from build123d import *

# Parameters (mm, degrees)
SKETCH2_R           = 6.281650674
SKETCH3_R           = 13.256970647
BOSS_EXTRUDE2_DEPTH = 93.98
FILLET1_R           = 5.08


with BuildPart() as part:
    # Sweep1: sweep along a curve in space
    with BuildLine() as sweep1_path:
        Line((-101.863707381, 710.985218526, -786.864459981), (-101.863707381, 710.985218526, -861.202210018))
        ThreePointArc((-101.863707381, 710.985218526, -861.202210018), (-107.071348812, 710.985218526, -873.774568588), (-119.643707381, 710.985218526, -878.982210018))
        Line((-119.643707381, 710.985218526, -878.982210018), (-194.958974291, 710.985218526, -878.982210018))
        ThreePointArc((-194.958974291, 710.985218526, -878.982210018), (-207.531332861, 710.985218526, -884.189851449), (-212.738974291, 710.985218526, -896.762210018))
        Line((-212.738974291, 710.985218526, -896.762210018), (-212.738974291, 710.985218526, -997.376214376))
    # Sketch2 → Sweep1 (sweep)
    with BuildSketch(Plane(origin=(-212.738974291, 710.985218526, -997.376214376), x_dir=(-1, 0, 0), z_dir=(0, 0, -1))):
        Circle(SKETCH2_R)
    sweep(path=sweep1_path.line)

    # Sketch3 → Boss-Extrude2 (add)
    with BuildSketch(Plane(origin=(0, 0, -997.376214376), x_dir=(-1, 0, 0), z_dir=(0, 0, -1))):
        with Locations((212.738974291, 710.985218526)):
            Circle(SKETCH3_R)
    extrude(amount=-BOSS_EXTRUDE2_DEPTH)

    # Fillet1
    fillet1_edges = [part.edges().sort_by_distance(p)[0] for p in [
        (-199.482003644, 710.985218526, -903.396214376),
        (-199.482003644, 710.985218526, -997.376214376),
    ]]
    fillet(fillet1_edges, radius=FILLET1_R)


solid = part.part
Check sheet for the modelled part. Datum: model origin and axes. Units: mm. A direction names the side the tool comes from. Give positions to 0.01 mm unless a question says otherwise; leave off trailing zeros. Order: outer loops, then holes, each group sorted by start corner. A loop starts at its lowest first (then second) coordinate and runs counter-clockwise, first axis right, second up. Notation, with made-up numbers: (64.25, 30.5) - (85.25, 30.5) arc R17 ccw to (85.25, 61.5) - close; hole circle Ø8 at (-11, 14.5). An arc over 180 degrees is marked (long way). Answer as CSV lines item,"result".
1. Scan lines: probe 1 along X at (y, z) = (710.5, -819); probe 2 along Z at (x, y) = (-205, 707.5); probe 3 along X at (y, z) = (714.5, -957). Record each from-to range of solid material in increasing order. Write a range as from..to.
Result sheet:
probe 1,"-108.13..-95.6"
probe 2,"-997.37..-903.41, -889.23..-876.06"
probe 3,"-225.52..-199.96"
2. Go/stop test with flat-tipped pins: P1, Ø8, axis at x = -120, y = 719, coming from the -Z side; P2, Ø6, axis at y = 708.5, z = -972.5, coming from the +X side; P3, Ø1.5, axis at y = 715.5, z = -839, coming from the -X side. Record where each tip stops, or that it passes through.
Result sheet:
P1,"z = -883.81"
P2,"x = -199.48"
P3,"x = -106.89"
3. Section check A-A (z = -972). Record the boundary of the cut face in (x, y).
Result sheet:
outline,"circle Ø26.51 at (-212.74, 710.99)"
4. Tool access check on faces 1 (the face through (-157.83, 708.58, -873.18)), 2 (the face through (-102, 711, -786.864)), 3 (the face through (-107.666, 708.579, -824.554)). Record the directions out of +Z, -Z, +X, -X, +Y, -Y that give a thin tool (end or side, any length) a straight path to the whole face; none if there is none.
Result sheet:
face 1,"none"
face 2,"+Z, +X, -X, +Y, -Y"
face 3,"+Z"
5. Mould release check, pull along Z, two halves, no side actions. Record for faces 4 (the face through (-213, 711, -997.376)), 5 (the face through (-209.865, 698.043, -950.973)), 6 (the face through (-206.463, 711.261, -900.126)): released by +Z, released by -Z, zero draft, split by the parting line, or undercut.
Result sheet:
face 4,"released by -Z"
face 5,"zero draft"
face 6,"undercut"
6. Section check B-B (x = -146). Record the boundary of the cut face in (y, z), then the cut area to 3 significant figures.
Result sheet:
outline,"circle Ø12.56 at (710.99, -878.98)"
area,"124 mm²"
